from build123d import *

# Parameters (mm, degrees)
FILLET1_R          = 2
CUT_EXTRUDE1_DEPTH = 5.44
CUT_EXTRUDE2_DEPTH = 5.19


with BuildPart() as part:
    # Sketch1 → Revolve1 (revolve)
    with BuildSketch(Plane.XY, mode=Mode.PRIVATE) as revolve1_sk:
        Polygon((-188.099626112, 0), (-188.099626112, 30), (-120.099626112, 30), (-120.099626112, 32.5), (9.900373888, 32.5), (9.900373888, 50), (38.900373888, 50), (38.900373888, 40), (118.900373888, 40), (118.900373888, 30), (177.400373888, 30), (177.400373888, 0), align=None)
    revolve(revolve1_sk.sketch.rotate(Axis((-188.099626112, 0, 0), (1, 0, 0)), 90), axis=Axis((-188.099626112, 0, 0), (1, 0, 0)))

    # Fillet1
    fillet1_edges = [part.edges().sort_by_distance(p)[0] for p in [
        (-188.099626112, 0, -30),
        (177.400373888, 0, -30),
    ]]
    fillet(fillet1_edges, radius=FILLET1_R)

    # Sketch2 → Cut-Extrude1 (cut)
    with BuildSketch(Plane(origin=(0, 32.5, 0), x_dir=(1, 0, 0), z_dir=(0, 1, 0))):
        with BuildLine():
            Line((-111.599626112, 6), (1.400373888, 6))
            ThreePointArc((1.400373888, 6), (7.400373888, 0), (1.400373888, -6))
            Line((1.400373888, -6), (-111.599626112, -6))
            ThreePointArc((-111.599626112, -6), (-117.599626112, 0), (-111.599626112, 6))
        make_face()
    extrude(amount=-CUT_EXTRUDE1_DEPTH, mode=Mode.SUBTRACT)

    # Sketch3 → Cut-Extrude2 (cut)
    with BuildSketch(Plane(origin=(0, 40, 0), x_dir=(1, 0, 0), z_dir=(0, 1, 0))):
        with BuildLine():
            Line((51.900373888, 8), (105.900373888, 8))
            ThreePointArc((105.900373888, 8), (113.900373888, 0), (105.900373888, -8))
            Line((105.900373888, -8), (51.900373888, -8))
            ThreePointArc((51.900373888, -8), (43.900373888, 0), (51.900373888, 8))
        make_face()
    extrude(amount=-CUT_EXTRUDE2_DEPTH, mode=Mode.SUBTRACT)


solid = part.part
Could you check a few things on this model? Use its own coordinates, in mm. A direction names the side the tool comes from. Give positions to 0.01 mm unless a question says otherwise; leave off trailing zeros. Order: outer loops, then holes, each group sorted by start corner. A loop starts at its lowest first (then second) coordinate and runs counter-clockwise, first axis right, second up.
1. Suppose I cut it at B-B (y = 0). List the corners of the cut face in (x, z) for me, plus the area to 3 significant figures.
2. Suppose I cut it at D-D (x = 129). List the corners of the cut face in (y, z) for me, plus the area to 3 significant figures.
3. Suppose I cut it at C-C (x = -46). List the corners of the cut face in (y, z) for me.
4. For faces 4 (the cylindrical face through (79.46, -1.76, -39.96)), 5 (the flat face through (177.4, 0, 0)), 6 (the flat face through (79, 34.81, 0)), 7 (the flat face through (9.9, 33, 1)), which set-ups out of +Z, -Z, +X, -X, +Y, -Y let a thin tool reach every point of the face, with its end or its side?
5. Will these pins go through, and if not, where does the flat tip stop? P1, Ø6, axis at x = -120, y = -4, coming from the +Z side; P2, Ø6, axis at x = -56, y = -16, coming from the -Z side; P3, Ø2.5, axis at x = -30.5, y = 30.5, coming from the +Z side.
6. We'd pull the mould along Z, two halves only. Please class faces 1 (the cylindrical face through (24.6, -15.02, 47.69)), 2 (the flat face through (-120.1, 29, -9)), 3 (the cylindrical face through (113.9, 37.44, -0.18)): pulls with the +Z half, pulls with the -Z half, needs draft (parallel to the pull), parting line crosses it, or undercut.
7. I need wall thicknesses on L1, parallel to Y at x = 159, z = 1.5; L2, parallel to X at y = 16, z = -31.5; L3, parallel to Y at x = 53, z = 1. Which ranges of each line are inside material? Lowest first, please.
Solved:
1. outline: (-188.1, -28) arc R2 ccw to (-186.1, -30) - (-120.1, -30) - (-120.1, -32.5) - (9.9, -32.5) - (9.9, -50) - (38.9, -50) - (38.9, -40) - (118.9, -40) - (118.9, -30) - (175.4, -30) arc R2 ccw to (177.4, -28) - (177.4, 28) arc R2 ccw to (175.4, 30) - (118.9, 30) - (118.9, 40) - (38.9, 40) - (38.9, 50) - (9.9, 50) - (9.9, 32.5) - (-120.1, 32.5) - (-120.1, 30) - (-186.1, 30) arc R2 ccw to (-188.1, 28) - close
1. area: 25,300 mm2
2. outline: circle Ø60 at (0, 0)
2. area: 2,830 mm2
3. outline: (27.06, -6) - (27.06, 6) - (31.94, 6) arc R32.5 ccw (long way) to (31.94, -6) - close
4. face 4: +X
4. face 5: +Z, -Z, +X, +Y, -Y
4. face 6: +Y
4. face 7: -X
5. P1: stops at z = 32.48
5. P2: stops at z = -29.79
5. P3: stops at z = 14.17
6. face 1: parting line crosses it
6. face 2: needs draft
6. face 3: undercut
7. L1: y = -29.96 to 29.96
7. L2: x = 9.9 to 118.9
7. L3: y = -39.99 to 34.81
